```python
from build123d import *

# Parameters (mm, degrees)
SKETCH1_W           = 20
SKETCH1_H           = 15
SKETCH1_R           = 1.55
BOSS_EXTRUDE1_DEPTH = 5
SKETCH2_W           = 20
SKETCH2_H           = 10
SKETCH2_R           = 0.791259191
BOSS_EXTRUDE2_DEPTH = 5
FILLET1_R           = 1


with BuildPart() as part:
    # Sketch1 → Boss-Extrude1 (new body)
    with BuildSketch(Plane.XY):
        Rectangle(SKETCH1_W, SKETCH1_H)
        with Locations((-5, 3.75)):
            Circle(SKETCH1_R, mode=Mode.SUBTRACT)
        with Locations(Location((5, 3.75, 0), (0, 0, 180))):
            Circle(SKETCH1_R, mode=Mode.SUBTRACT)
        with Locations((5, -3.75)):
            Circle(SKETCH1_R, mode=Mode.SUBTRACT)
        with Locations(Location((-5, -3.75, 0), (0, 0, 180))):
            Circle(SKETCH1_R, mode=Mode.SUBTRACT)
    extrude(amount=BOSS_EXTRUDE1_DEPTH)

    # Sketch2 → Boss-Extrude2 (add)
    with BuildSketch(Plane(origin=(0, 7.5, 0), x_dir=(1, 0, 0), z_dir=(0, 1, 0))):
        Rectangle(SKETCH2_W, SKETCH2_H)
        with Locations(Location((-5, 2.5, 0), (0, 0, 270))):
            Circle(SKETCH2_R, mode=Mode.SUBTRACT)
        with Locations(Location((5, 2.5, 0), (0, 0, 90))):
            Circle(SKETCH2_R, mode=Mode.SUBTRACT)
    extrude(amount=BOSS_EXTRUDE2_DEPTH)

    # Fillet1
    fillet1_edges = [part.edges().sort_by_distance(p)[0] for p in [
        (-10, 7.5, -2.5),
        (10, 7.5, -2.5),
        (0, 7.5, -5),
        (0, 7.5, 0),
        (10, 0, 0),
        (0, -7.5, 0),
        (-10, 0, 0),
        (10, -7.5, 2.5),
        (-10, -7.5, 2.5),
    ]]
    fillet(fillet1_edges, radius=FILLET1_R)


solid = part.part
```
Geometry: final body of the model. Coordinates: model frame, mm. A direction names the side the tool comes from. Coordinates: 2 decimals unless noted, no trailing zeros. Order: outer loops, then holes, each group sorted by start corner. A loop starts at its lowest first (then second) coordinate and runs counter-clockwise, first axis right, second up. Notation, with made-up numbers: (-39, 87) -> (19, 87) arc R32 cw to (19, 118) -> close; hole circle Ø4 at (-34, 11.5). An arc over 180 degrees is marked (long way). Use CSV: the item, a comma, the result in double quotes.
1) Section B-B on y = 3.75. Output: boundary loops of the cut face in (x, z), then the cut area to 3 significant figures.
Findings:
outline,"(-10, 1) arc R1 ccw to (-9, 0) -> (-6.55, 0) -> (-6.55, 5) -> (-10, 5) -> close; (-3.45, 0) -> (3.45, 0) -> (3.45, 5) -> (-3.45, 5) -> close; (6.55, 0) -> (9, 0) arc R1 ccw to (10, 1) -> (10, 5) -> (6.55, 5) -> close"
area,"68.6 mm^2"
2) Section C-C on x = -5. Output: boundary loops of the cut face in (y, z).
Findings:
outline,"(-7.5, 1) arc R1 ccw to (-6.5, 0) -> (-5.3, 0) -> (-5.3, 5) -> (-7.5, 5) -> close; (-2.2, 0) -> (2.2, 0) -> (2.2, 5) -> (-2.2, 5) -> close; (5.3, 0) -> (6.5, 0) arc R1 cw to (7.5, -1) -> (7.5, -1.71) -> (12.5, -1.71) -> (12.5, 5) -> (5.3, 5) -> close; (7.5, -4) arc R1 ccw to (8.5, -5) -> (12.5, -5) -> (12.5, -3.29) -> (7.5, -3.29) -> close"
3) Section A-A on z = -2.5. Output: boundary loops of the cut face in (x, y).
Findings:
outline,"(-10, 8.5) arc R1 ccw to (-9, 7.5) -> (-5.79, 7.5) -> (-5.79, 12.5) -> (-10, 12.5) -> close; (-4.21, 7.5) -> (4.21, 7.5) -> (4.21, 12.5) -> (-4.21, 12.5) -> close; (5.79, 7.5) -> (9, 7.5) arc R1 ccw to (10, 8.5) -> (10, 12.5) -> (5.79, 12.5) -> close"
4) Access query for faces 1 (the flat face through (0, 0, 0)), 2 (the cylindrical face through (9.715, -7.199, 3.028)), 3 (the cylindrical face through (-9.715, 7.801, -3.028)). Directions: +Z, -Z, +X, -X, +Y, -Y. A direction counts if a zero-diameter tool reaches every point of the face in a straight line with its end or side. Return the directions, or none.
Findings:
face 1,"-Z, +X, -X, -Y"
face 2,"+Z, -Z, +X, -Y"
face 3,"-Z, -X, -Y"
5) Pin query (flat end, axial travel): pin 1 Ø2 at (x, z) = (5, -2.5) entering from -Y; pin 2 Ø6 at (x, z) = (7, -1) entering from -Y; pin 3 Ø4 at (x, y) = (0, -0.5) entering from -Z; pin 4 Ø1.9 at (x, y) = (5, -3.75) entering from +Z. Return the tip coordinate at first contact, or that it passes through.
Findings:
pin 1,"stops at y = 7.5"
pin 2,"stops at y = -7.5"
pin 3,"stops at z = 0"
pin 4,"passes through"
6) Mould query, pull axis Z, two halves, no side actions, for faces 4 (the flat face through (0, 2, 5)), 5 (the cylindrical face through (9.715, 0.091, 0.301)), 6 (the cylindrical face through (5.772, 9.965, -2.328)). Classes: +Z half, -Z half, draft (parallel to the pull), parting line (faces both ways), or undercut.
Findings:
face 4,"+Z half"
face 5,"-Z half"
face 6,"undercut"
7) Line query: line 1 (Y direction, x = -5, z = 3.1); line 2 (X direction, y = 9.9, z = -2.5); line 3 (Z direction, x = 5, y = 11). Output: solid intervals per line, ascending.
Findings:
line 1,"y = -7.5 to -5.3, -2.2 to 2.2, 5.3 to 12.5"
line 2,"x = -10 to -5.79, -4.21 to 4.21, 5.79 to 10"
line 3,"z = -5 to -3.29, -1.71 to 5"
8) Section D-D on z = 3. Output: boundary loops of the cut face in (x, y), then the cut area to 3 significant figures.
Findings:
outline,"(-10, -6.5) arc R1 ccw to (-9, -7.5) -> (9, -7.5) arc R1 ccw to (10, -6.5) -> (10, 12.5) -> (-10, 12.5) -> close; hole circle Ø3.1 at (-5, -3.75); hole circle Ø3.1 at (-5, 3.75); hole circle Ø3.1 at (5, -3.75); hole circle Ø3.1 at (5, 3.75)"
area,"369 mm^2"
